from build123d import *

# Parameters (mm, degrees)
SKETCH1_W           = 800
SKETCH1_H           = 800
BOSS_EXTRUDE1_DEPTH = 15
SKETCH2_R           = 5
CUT_EXTRUDE1_DEPTH  = 15
SKETCH4_R           = 8
CUT_EXTRUDE2_DEPTH  = 15
SKETCH5_R           = 10
CUT_EXTRUDE3_DEPTH  = 567.480361531


with BuildPart() as part:
    # Sketch1 → Boss-Extrude1 (new, symmetric)
    with BuildSketch(Plane(origin=(0, 0, 0), x_dir=(1, 0, 0), z_dir=(0, 1, 0))):
        Rectangle(SKETCH1_W, SKETCH1_H)
    extrude(amount=BOSS_EXTRUDE1_DEPTH, both=True)

    # Sketch2 → Cut-Extrude1 (cut)
    with BuildSketch(Plane(origin=(0, 15, 0), x_dir=(1, 0, 0), z_dir=(0, 1, 0))):
        with Locations(Location((0, 188.5, 0), (0, 0, 270))):
            Circle(SKETCH2_R)
        with Locations(Location((188.5, 0, 0), (0, 0, 270))):
            Circle(SKETCH2_R)
        with Locations(Location((0, -188.5, 0), (0, 0, 90))):
            Circle(SKETCH2_R)
        with Locations(Location((-188.5, 0, 0), (0, 0, 90))):
            Circle(SKETCH2_R)
        with Locations(Location((133.289628254, 133.289628254, 0), (0, 0, 270))):
            Circle(SKETCH2_R)
        with Locations(Location((-133.289628254, -133.289628254, 0), (0, 0, 90))):
            Circle(SKETCH2_R)
        with Locations(Location((133.289628254, -133.289628254, 0), (0, 0, 270))):
            Circle(SKETCH2_R)
        with Locations(Location((-133.289628254, 133.289628254, 0), (0, 0, 90))):
            Circle(SKETCH2_R)
    extrude(amount=-CUT_EXTRUDE1_DEPTH, mode=Mode.SUBTRACT)

    # Sketch4 → Cut-Extrude2 (cut)
    with BuildSketch(Plane(origin=(0, 15, 0), x_dir=(1, 0, 0), z_dir=(0, 1, 0))):
        with Locations(Location((0, 345, 0), (0, 0, 270))):
            Circle(SKETCH4_R)
        with Locations(Location((132.025784166, 318.738438716, 0), (0, 0, 270))):
            Circle(SKETCH4_R)
        with Locations(Location((243.951839509, 243.951839509, 0), (0, 0, 270))):
            Circle(SKETCH4_R)
        with Locations(Location((318.738438716, 132.025784166, 0), (0, 0, 270))):
            Circle(SKETCH4_R)
        with Locations(Location((345, 0, 0), (0, 0, 270))):
            Circle(SKETCH4_R)
        with Locations(Location((318.738438716, -132.025784166, 0), (0, 0, 270))):
            Circle(SKETCH4_R)
        with Locations(Location((243.951839509, -243.951839509, 0), (0, 0, 270))):
            Circle(SKETCH4_R)
        with Locations(Location((132.025784166, -318.738438716, 0), (0, 0, 270))):
            Circle(SKETCH4_R)
        with Locations(Location((0, -345, 0), (0, 0, 270))):
            Circle(SKETCH4_R)
        with Locations(Location((-132.025784166, -318.738438716, 0), (0, 0, 270))):
            Circle(SKETCH4_R)
        with Locations(Location((-243.951839509, -243.951839509, 0), (0, 0, 270))):
            Circle(SKETCH4_R)
        with Locations(Location((-318.738438716, -132.025784166, 0), (0, 0, 270))):
            Circle(SKETCH4_R)
        with Locations(Location((-345, 0, 0), (0, 0, 270))):
            Circle(SKETCH4_R)
        with Locations(Location((-318.738438716, 132.025784166, 0), (0, 0, 270))):
            Circle(SKETCH4_R)
        with Locations(Location((-243.951839509, 243.951839509, 0), (0, 0, 270))):
            Circle(SKETCH4_R)
        with Locations(Location((-132.025784166, 318.738438716, 0), (0, 0, 270))):
            Circle(SKETCH4_R)
    extrude(amount=-CUT_EXTRUDE2_DEPTH, mode=Mode.SUBTRACT)

    # Sketch5 → Cut-Extrude3 (cut, through all)
    with BuildSketch(Plane(origin=(0, 15, 0), x_dir=(1, 0, 0), z_dir=(0, 1, 0))):
        with Locations(Location((-370, 370, 0), (0, 0, 270))):
            Circle(SKETCH5_R)
        with Locations(Location((370, 370, 0), (0, 0, 90))):
            Circle(SKETCH5_R)
        with Locations(Location((370, -370, 0), (0, 0, 270))):
            Circle(SKETCH5_R)
        with Locations(Location((-370, -370, 0), (0, 0, 90))):
            Circle(SKETCH5_R)
    extrude(amount=-CUT_EXTRUDE3_DEPTH, mode=Mode.SUBTRACT)


solid = part.part
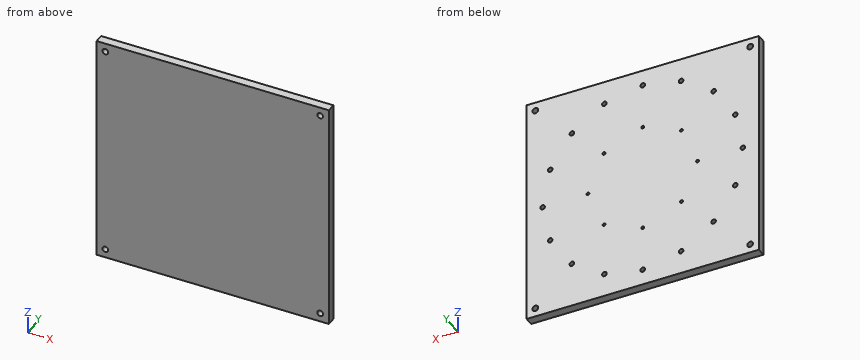
Source: CAD feature listing. Evaluate the final solid. Frame: model axes, mm. Give positions to 0.01 mm unless a question says otherwise; leave off trailing zeros. Write each loop counter-clockwise with the first axis right and the second up, starting at its lowest first coordinate (ties: lowest second). Pieces come first, ordered by that corner, then holes. Notation, with made-up numbers: M 24.25,27 L 71.25,27 A19 ccw 71.25,50 Z; hole C 37,-5.5 d5. An arc over 180 degrees is marked long. Return JSON: item names as keys, results as strings. Group by question number.
1) Pin query (flat end, axial travel): P1, Ø16, axis at x = -370, z = 370, coming from the -Y side; P2, Ø13, axis at x = 319, z = -131, coming from the +Y side. Return the tip coordinate at first contact, or that it passes through.
2) Cut plane A-A, the plane x = 370. Output: boundary loops of the cut face in (y, z), plus the area to 3 significant figures.
3) Material intervals for line 1 along Z through (x, y) = (-362, -11.75); line 2 along X through (y, z) = (13, 134.5); line 3 along Z through (x, y) = (-188.5, 12), sorted ascending. Write a range as [from, to].
4) Cut plane B-B, the plane z = 370. Output: boundary loops of the cut face in (x, y), plus the area to 3 significant figures.
Recorded:
{
 "1": {"P1": "passes through", "P2": "stops at y = 0"},
 "2": {"outline": "M -15,-400 L 15,-400 L 15,-380 L -15,-380 Z; M -15,-360 L 15,-360 L 15,360 L -15,360 Z; M -15,380 L 15,380 L 15,400 L -15,400 Z", "area": "22,800 mm²"},
 "3": {"line 1": "z = [-400, -376], [-364, 364], [376, 400]", "line 2": "x = [-400, -326.35], [-311.13, -138.14], [-128.44, 128.44], [138.14, 311.13], [326.35, 400]", "line 3": "z = [-400, -5], [5, 400]"},
 "4": {"outline": "M -400,-15 L -380,-15 L -380,15 L -400,15 Z; M -360,-15 L 360,-15 L 360,15 L -360,15 Z; M 380,-15 L 400,-15 L 400,15 L 380,15 Z", "area": "22,800 mm²"}
}
